Model file for the job. Use its own axes, mm. Coordinates: 2 decimals unless noted, no trailing zeros. Order: outer loops, then holes, each group sorted by start corner. A loop starts at its lowest first (then second) coordinate and runs counter-clockwise, first axis right, second up.
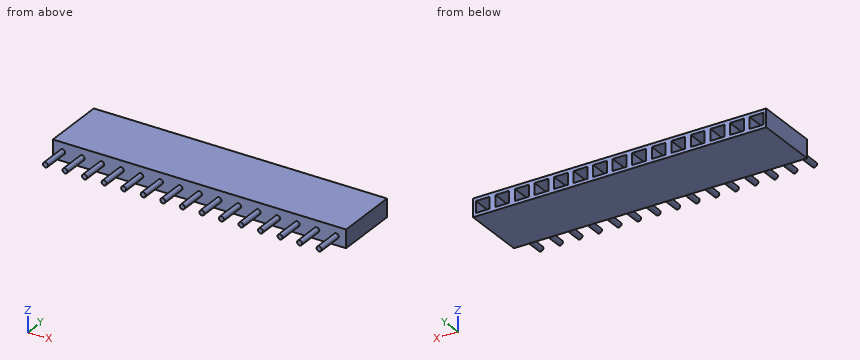
from build123d import *

# Parameters (mm, degrees)
ESQUISSE1_W                = 2.54
ESQUISSE1_H                = 2.35
BOSS_EXTRU_1_DEPTH         = 8.35
ESQUISSE3_W                = 1.8
ESQUISSE3_H                = 1.5
ENL_V_MAT_EXTRU_1_DEPTH    = 5.5
ESQUISSE2_R                = 0.325
BOSS_EXTRU_2_DEPTH         = 3.5
ESQUISSE4_R                = 0.325
ENL_V_MAT_EXTRU_3_DEPTH    = 2
R_P_TITION_LIN_AIRE1_COUNT = 15
R_P_TITION_LIN_AIRE1_PITCH = 2.54


with BuildPart() as part:
    # Esquisse1 → Boss.-Extru.1 (new body)
    with BuildSketch(Plane(origin=(0, 0, 0), x_dir=(1, 0, 0), z_dir=(0, 1, 0))):
        with Locations((1.27, 1.175)):
            Rectangle(ESQUISSE1_W, ESQUISSE1_H)
    boss_extru_1 = extrude(amount=BOSS_EXTRU_1_DEPTH)

    # Esquisse3 → Enlèv. mat.-Extru.1 (cut)
    with BuildSketch(Plane(origin=(0, 8.35, 0), x_dir=(1, 0, 0), z_dir=(0, 1, 0))):
        with Locations((1.27, 1.175)):
            Rectangle(ESQUISSE3_W, ESQUISSE3_H)
    enl_v_mat_extru_1 = extrude(amount=-ENL_V_MAT_EXTRU_1_DEPTH, mode=Mode.SUBTRACT)

    # Esquisse2 → Boss.-Extru.2 (add)
    with BuildSketch(Plane.XZ):
        with Locations(Location((1.27, -1.175, 0), (0, 0, 270))):
            Circle(ESQUISSE2_R)
    boss_extru_2 = extrude(amount=BOSS_EXTRU_2_DEPTH)

    # Esquisse4 → Enlèv. mat.-Extru.3 (cut)
    with BuildSketch(Plane(origin=(0, 2.85, 0), x_dir=(1, 0, 0), z_dir=(0, 1, 0))):
        with Locations(Location((1.27, 1.175, 0), (0, 0, 90))):
            Circle(ESQUISSE4_R)
    enl_v_mat_extru_3 = extrude(amount=-ENL_V_MAT_EXTRU_3_DEPTH, mode=Mode.SUBTRACT)

    # Répétition linéaire1: Boss.-Extru.1, Enlèv. mat.-Extru.1, Boss.-Extru.2, Enlèv. mat.-Extru.3 ×15
    with Locations(*[(i * R_P_TITION_LIN_AIRE1_PITCH, 0, 0) for i in range(1, R_P_TITION_LIN_AIRE1_COUNT)]):
        add(boss_extru_1)
        add(enl_v_mat_extru_1, mode=Mode.SUBTRACT)
        add(boss_extru_2)
        add(enl_v_mat_extru_3, mode=Mode.SUBTRACT)


solid = part.part
Q1. Drop a flat-ended pin along its axis: P1, Ø0.5, axis at x = 14, z = -1, coming from the +Y side. Give the stop position or say it passes through.
Established:
P1: stops at y = 2.85
Q2. Cut at A-A, the plane x = 29.21. List the corners of the cut face in (y, z) (3 decimals).
Established:
outline: (-3.5, -1.5) - (0, -1.5) - (0, -2.35) - (8.35, -2.35) - (8.35, -1.925) - (2.85, -1.925) - (2.85, -1.5) - (0.85, -1.5) - (0.85, -0.85) - (2.85, -0.85) - (2.85, -0.425) - (8.35, -0.425) - (8.35, 0) - (0, 0) - (0, -0.85) - (-3.5, -0.85) - close
Q3. Cut at B-B, the plane y = 5.25. Count the separate pieces of the cut face and the enclosed holes in it, plus the area to 3 significant figures.
Established:
separate pieces: 1
enclosed holes: 15
area: 49.0 mm2
Q4. Probe line 1 (Z direction, x = 6, y = 8) (3 decimals); line 2 (Z direction, x = 21.59, y = 2.45); line 3 (Y direction, x = 15.5, z = -2). List the from-to ranges inside material, lowest first.
Established:
line 1: z = -2.35 to -1.925, -0.425 to 0
line 2: z = -2.35 to -1.5, -0.85 to 0
line 3: y = 0 to 8.35
